The model under review builds one solid part; all positions refer to its coordinate system, in mm. Face numbers are marked on the shaded views. A direction names the side the tool comes from. Round coordinates to 2 decimals unless told otherwise and drop trailing zeros. Loops run counter-clockwise (first coordinate to the right, second up) from the corner with the lowest first, then second, coordinate; pieces in that order, holes last. Notation, with made-up numbers: M -15.75,2 L 23.25,2 A17 cw 23.25,19 Z; hole C 84,-15 d8. An arc over 180 degrees is marked long. Return JSON: item names as keys, results as strings. Group by question number.
Q1. Consider section B-B (x = 0). State the section outline as (y, z) points, and give its area (3 significant figures).
Q2. Clearance check with flat-ended pins moving along their axes: pin 1 Ø1 at (y, z) = (3.5, 9.5) entering from -X; pin 2 Ø3 at (y, z) = (6.5, 6.5) entering from +X; pin 3 Ø1 at (y, z) = (2.5, 2.5) entering from -X. State where each tip first meets the part, or that it passes through.
Q3. Consider section C-C (z = 7). State the section outline as (x, y) points.
Q4. Consider section D-D (z = 1.25). State the section outline as (x, y) points.
Q5. For the marked faces 5 and 6, list the 3-axis set-ups (+Z, -Z, +X, -X, +Y, -Y) from which the entire face can be reached by the end or side of a thin tool; tool diameter is ignored.
Q6. Consider section A-A (y = 6.25). State the section outline as (x, z) points, and give its area (3 significant figures).
Q7. Draft analysis for pull direction Z (two halves, no side actions). For the marked faces 1, 2, 3 and 4, state which applies: pulls with the +Z half, pulls with the -Z half, needs draft (parallel to the pull), parting line crosses it, or undercut.
Q8. To check wall thickness, follow line 1 along X through (y, z) = (4.25, 4.75); line 2 along X through (y, z) = (15.3, 6); line 3 along X through (y, z) = (10.5, 6.5). State the ranges of each line that lie inside material, in increasing order.
from build123d import *

# Parameters (mm, degrees)
ESTRUSIONE_ESTRUSIONE1_DEPTH = 12
SCHIZZO2_R                   = 2
TAGLIO_ESTRUSIONE1_DEPTH     = 32.786381776
SCHIZZO3_R                   = 3
TAGLIO_ESTRUSIONE2_DEPTH     = 2.5
ESTRUSIONE_ESTRUSIONE2_START = -1.85
ESTRUSIONE_ESTRUSIONE2_DEPTH = 1.85
ESTRUSIONE_ESTRUSIONE3_DEPTH = 1.85


with BuildPart() as part:
    # Schizzo1 → Estrusione-Estrusione1 (new body)
    with BuildSketch(Plane.XY):
        with BuildLine():
            Line((21, 17.1), (-21, 17.1))
            Line((-21, 17.1), (-21, 0))
            Line((-21, 0), (-12.1, 0))
            ThreePointArc((-12.1, 0), (0, 12.1), (12.1, 0))
            Line((12.1, 0), (21, 0))
            Line((21, 0), (21, 17.1))
        make_face()
        Polygon((-21, 17.1), (-23.95754717, 0), (-21, 0), align=None)
        Polygon((21, 0), (23.95754717, 0), (21, 17.1), align=None)
    extrude(amount=ESTRUSIONE_ESTRUSIONE1_DEPTH)

    # Schizzo2 → Taglio-Estrusione1 (cut, through all)
    with BuildSketch(Plane.XZ):
        with Locations((-18.028773585, 6)):
            Circle(SCHIZZO2_R)
        with Locations((18.028773585, 6)):
            Circle(SCHIZZO2_R)
    extrude(amount=-TAGLIO_ESTRUSIONE1_DEPTH, mode=Mode.SUBTRACT)

    # Schizzo3 → Taglio-Estrusione2 (cut)
    with BuildSketch(Plane(origin=(0, 17.1, 0), x_dir=(1, 0, 0), z_dir=(0, 1, 0))):
        with Locations(Location((-18.028773585, -6, 0), (0, 0, 180))):
            Circle(SCHIZZO3_R)
        with Locations(Location((18.028773585, -6, 0), (0, 0, 180))):
            Circle(SCHIZZO3_R)
    extrude(amount=-TAGLIO_ESTRUSIONE2_DEPTH, mode=Mode.SUBTRACT)

    # Schizzo4 → Estrusione-Estrusione2 (add)
    with BuildSketch(Plane.XY.offset(12).offset(ESTRUSIONE_ESTRUSIONE2_START)):
        with BuildLine():
            ThreePointArc((-10.5, 0), (0, 10.5), (10.5, 0))
            Line((10.5, 0), (12.1, 0))
            ThreePointArc((12.1, 0), (0, 12.1), (-12.1, 0))
            Line((-12.1, 0), (-10.5, 0))
        make_face()
    extrude(amount=ESTRUSIONE_ESTRUSIONE2_DEPTH)

    # Schizzo5 → Estrusione-Estrusione3 (add)
    with BuildSketch(Plane(origin=(0, 0, 0), x_dir=(-1, 0, 0), z_dir=(0, 0, -1))):
        with BuildLine():
            Line((10.5, 0), (12.1, 0))
            ThreePointArc((12.1, 0), (0, 12.1), (-12.1, 0))
            Line((-12.1, 0), (-10.5, 0))
            ThreePointArc((-10.5, 0), (0, 10.5), (10.5, 0))
        make_face()
    extrude(amount=-ESTRUSIONE_ESTRUSIONE3_DEPTH)


solid = part.part
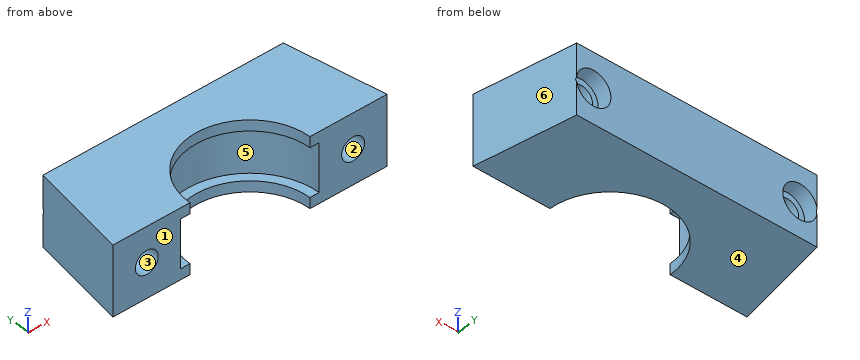
Values:
{
 "1": {"outline": "M 10.5,0 L 17.1,0 L 17.1,12 L 10.5,12 L 10.5,10.15 L 12.1,10.15 L 12.1,1.85 L 10.5,1.85 Z", "area": "65.9 mm2"},
 "2": {"pin 1": "stops at x = -23.44", "pin 2": "stops at x = 23.09", "pin 3": "stops at x = -23.61"},
 "3": {"outline": "M -23.96,0 L -19.76,0 L -19.76,14.6 L -20.86,14.6 L -20.86,17.1 L -21,17.1 Z; M -16.3,0 L -12.1,0 A12.1 cw 12.1,0 L 16.3,0 L 16.3,14.6 L 15.2,14.6 L 15.2,17.1 L -15.2,17.1 L -15.2,14.6 L -16.3,14.6 Z; M 19.76,0 L 23.96,0 L 21,17.1 L 20.86,17.1 L 20.86,14.6 L 19.76,14.6 Z"},
 "4": {"outline": "M -23.96,0 L -10.5,0 A10.5 cw 10.5,0 L 23.96,0 L 21,17.1 L -21,17.1 Z"},
 "5": {"face 5": "-Y", "face 6": "+Z, -Z, +X, +Y"},
 "6": {"outline": "M -22.88,0 L -8.44,0 L -8.44,1.85 L -10.36,1.85 L -10.36,10.15 L -8.44,10.15 L -8.44,12 L -22.88,12 Z; M 8.44,0 L 22.88,0 L 22.88,12 L 8.44,12 L 8.44,10.15 L 10.36,10.15 L 10.36,1.85 L 8.44,1.85 Z; hole C -18.03,6 d4; hole C 18.03,6 d4", "area": "289 mm2"},
 "7": {"face 1": "needs draft", "face 2": "undercut", "face 3": "undercut", "face 4": "pulls with the -Z half"},
 "8": {"line 1": "x = -23.22 to -19.59, -16.47 to -11.33, 11.33 to 16.47, 19.59 to 23.22", "line 2": "x = -21.31 to -21.03, -15.03 to 15.03, 21.03 to 21.31", "line 3": "x = -22.14 to -19.97, -16.09 to -6.01, 6.01 to 16.09, 19.97 to 22.14"}
}
